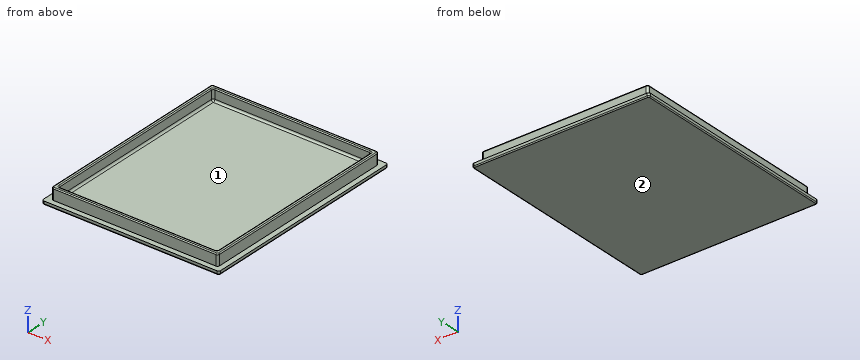
from build123d import *

# Parameters (mm, degrees)
SKETCH1_W           = 90
SKETCH1_H           = 108
BOSS_EXTRUDE1_DEPTH = 1.8
SKETCH2_W           = 84.7
SKETCH2_H           = 102.7
SKETCH2_W_2         = 80.7
SKETCH2_H_2         = 98.7
BOSS_EXTRUDE2_DEPTH = 5.8
FILLET1_R           = 1
FILLET2_R           = 0.5


with BuildPart() as part:
    # Sketch1 → Boss-Extrude1 (new body)
    with BuildSketch(Plane.XY):
        Rectangle(SKETCH1_W, SKETCH1_H)
    extrude(amount=BOSS_EXTRUDE1_DEPTH)

    # Sketch2 → Boss-Extrude2 (add)
    with BuildSketch(Plane.XY.offset(1.8)):
        Rectangle(SKETCH2_W, SKETCH2_H)
        Rectangle(SKETCH2_W_2, SKETCH2_H_2, mode=Mode.SUBTRACT)
    extrude(amount=BOSS_EXTRUDE2_DEPTH)

    # Fillet1
    fillet1_edges = [part.edges().sort_by_distance(p)[0] for p in [
        (-40.35, 0, 1.8),
        (0, -49.35, 1.8),
        (40.35, 0, 1.8),
        (0, 49.35, 1.8),
        (-42.35, 51.35, 4.7),
        (-42.35, -51.35, 4.7),
        (42.35, -51.35, 4.7),
        (42.35, 51.35, 4.7),
        (-40.35, -49.35, 4.7),
        (40.35, -49.35, 4.7),
        (40.35, 49.35, 4.7),
        (-40.35, 49.35, 4.7),
        (45, -54, 0.9),
        (-45, -54, 0.9),
        (-45, 54, 0.9),
        (45, 54, 0.9),
    ]]
    fillet(fillet1_edges, radius=FILLET1_R)

    # Fillet2
    fillet2_edges = [part.edges().sort_by_distance(p)[0] for p in [
        (0, 49.35, 7.6),
        (40.35, 0, 7.6),
        (0, -49.35, 7.6),
        (-40.35, 0, 7.6),
        (0, -54, 0),
        (45, 0, 0),
        (-45, 0, 0),
        (0, 54, 0),
        (44.707106781, 53.707106781, 0),
        (44.707106781, -53.707106781, 0),
        (-44.707106781, 53.707106781, 0),
        (-44.707106781, -53.707106781, 0),
        (-42.35, 0, 7.6),
        (0, 51.35, 7.6),
        (0, -51.35, 7.6),
        (42.35, 0, 7.6),
        (42.057106781, 51.057106781, 7.6),
        (-42.057106781, -51.057106781, 7.6),
        (42.057106781, -51.057106781, 7.6),
        (-42.057106781, 51.057106781, 7.6),
        (40.057106781, -49.057106781, 7.6),
        (40.057106781, 49.057106781, 7.6),
        (-40.057106781, 49.057106781, 7.6),
        (-40.057106781, -49.057106781, 7.6),
    ]]
    fillet(fillet2_edges, radius=FILLET2_R)


solid = part.part
The model under review builds one solid part; all positions refer to its coordinate system, in mm. Face numbers are marked on the shaded views. Round coordinates to 2 decimals unless told otherwise and drop trailing zeros. Loops run counter-clockwise (first coordinate to the right, second up) from the corner with the lowest first, then second, coordinate; pieces in that order, holes last. Notation, with made-up numbers: (56, 50.25) -> (115, 50.25) arc R16 cw to (115, 67.25) -> close; hole circle Ø7 at (76.25, 16). An arc over 180 degrees is marked (long way). Write item = value, one per line. Start each with the question number.
Item 1: Mouldability with a two-part tool opening along Y and no side actions: class the marked faces 1 and 2 as released by +Y, released by -Y, zero draft, split by the parting line, or undercut.
Item 2: Take a section at C-C on y = -19. Give the boundary of the cut face in (x, z), plus the area to 3 significant figures.
Item 3: To check wall thickness, follow L1, parallel to Y at x = -6, z = 5.5; L2, parallel to X at y = -41.5, z = 6.25; L3, parallel to Y at x = 15.5, z = 7.25. State the ranges of each line that lie inside material, in increasing order.
Item 4: Insertion check: pin 1 (1.3 mm diameter, centred on x = 3, z = 5.5, fed in from +Y); pin 2 (2.5 mm diameter, centred on y = -7.5, z = 3.5, fed in from -X); pin 3 (4.5 mm diameter, centred on x = 2.5, z = 5.5, fed in from -Y). Each pin has a flat end and moves straight along its axis. Give the tip position at first contact, or say it passes through.
Item 5: Take a section at B-B on x = -7. Give the boundary of the cut face in (y, z), plus the area to 3 significant figures.
Item 6: Take a section at A-A on z = 4. Give the boundary of the cut face in (x, y).
Result:
q1.face_1 = undercut
q1.face_2 = zero draft
q2.outline = (-45, 0.5) arc R0.5 ccw to (-44.5, 0) -> (44.5, 0) arc R0.5 ccw to (45, 0.5) -> (45, 1.8) -> (42.35, 1.8) -> (42.35, 7.1) arc R0.5 ccw to (41.85, 7.6) -> (40.85, 7.6) arc R0.5 ccw to (40.35, 7.1) -> (40.35, 2.8) arc R1 cw to (39.35, 1.8) -> (-39.35, 1.8) arc R1 cw to (-40.35, 2.8) -> (-40.35, 7.1) arc R0.5 ccw to (-40.85, 7.6) -> (-41.85, 7.6) arc R0.5 ccw to (-42.35, 7.1) -> (-42.35, 1.8) -> (-45, 1.8) -> close
q2.area = 185 mm²
q3.L1 = -51.35 to -49.35, 49.35 to 51.35
q3.L2 = -42.35 to -40.35, 40.35 to 42.35
q3.L3 = -51.33 to -49.37, 49.37 to 51.33
q4.pin_1 = 51.35
q4.pin_2 = -42.35
q4.pin_3 = -51.35
q5.outline = (-54, 0.5) arc R0.5 ccw to (-53.5, 0) -> (53.5, 0) arc R0.5 ccw to (54, 0.5) -> (54, 1.8) -> (51.35, 1.8) -> (51.35, 7.1) arc R0.5 ccw to (50.85, 7.6) -> (49.85, 7.6) arc R0.5 ccw to (49.35, 7.1) -> (49.35, 2.8) arc R1 cw to (48.35, 1.8) -> (-48.35, 1.8) arc R1 cw to (-49.35, 2.8) -> (-49.35, 7.1) arc R0.5 ccw to (-49.85, 7.6) -> (-50.85, 7.6) arc R0.5 ccw to (-51.35, 7.1) -> (-51.35, 1.8) -> (-54, 1.8) -> close
q5.area = 218 mm²
q6.outline = (-42.35, -50.35) arc R1 ccw to (-41.35, -51.35) -> (41.35, -51.35) arc R1 ccw to (42.35, -50.35) -> (42.35, 50.35) arc R1 ccw to (41.35, 51.35) -> (-41.35, 51.35) arc R1 ccw to (-42.35, 50.35) -> close; hole (-40.35, -48.35) arc R1 ccw to (-39.35, -49.35) -> (39.35, -49.35) arc R1 ccw to (40.35, -48.35) -> (40.35, 48.35) arc R1 ccw to (39.35, 49.35) -> (-39.35, 49.35) arc R1 ccw to (-40.35, 48.35) -> close
